For this review, take the finished solid that the model builds, in its own axes (mm). Give positions to 0.01 mm unless a question says otherwise; leave off trailing zeros. Loops run counter-clockwise (first coordinate to the right, second up) from the corner with the lowest first, then second, coordinate; pieces in that order, holes last. Notation, with made-up numbers: (46, 27.5) - (78, 27.5) arc R17 cw to (78, 48.5) - close; hole circle Ø9 at (56, 29). An arc over 180 degrees is marked (long way). Put each result on its own line as item: value.
Autodesk Fusion 360 part; units mm, degrees
sketch "Skizze1" plane through (0, 0, 0) normal (0, 0, 1) x (1, 0, 0)
  line L0 (-2.5, 19.7043) -> (-8.5, 19.7043)
  line L1 (-8.5, 19.7043) -> (-8.5, -52.5)
  line L2 (-8.5, -52.5) -> (-2.5, -52.5)
  line L3 (-2.5, -52.5) -> (-2.5, -35.8)
  line L4 (-2.5, -35.8) -> (0, -38.3)
  line L5 (0, -38.3) -> (0, 38.3)
  line L6 (0, 38.3) -> (-2.5, 35.8)
  line L7 (-2.5, 35.8) -> (-2.5, 19.7043)
  line L8 (-2.5, 35.8) -> (-8.5, 29.8)
  line L9 (-8.5, 29.8) -> (-8.5, 19.7043)
  line L10 (-0.5, 37.8) -> (-0.25, 37.8)
  line L11 (-0.25, 37.8) -> (0, 37.55)
  line L12 (0, 0) -> (7.5514, 0) construction
  line L13 (-0.5, -37.8) -> (-0.25, -37.8)
  line L14 (-0.25, -37.8) -> (0, -37.55)
  dimension "d1" = 45
  dimension "d2" = 2.5
  dimension "d6" = 52.5
  dimension "d31" = 8.5
  dimension "d33" = 16.7
  dimension "d34" = 0.25
  dimension "d36" = 0.25
  dimension "d37" = 82.3
extrude "Extrusion1" add sketch "Skizze1" along normal blind 76 contours L0 L1 L2 L3 L4 L5 L6 L7 L10 L11 L13 L14 | L0 L7 L8 L9
sketch "Skizze2" plane through (0, 0, 0) normal (1, 0, 0) x (0, 1, 0)
  line L0 (-37.55, 0) -> (37.55, 0)
  line L1 (37.55, 76) -> (-37.55, 76)
  line L2 (0, 38) -> (-32.5, 38) construction
  circle A0 centre (-12.5, 38) radius 2
  circle A1 centre (-32.5, 38) radius 2
  circle A2 centre (-22.5, 48) radius 2
  circle A3 centre (-22.5, 28) radius 2
  line L3 (-32.5, 38) -> (-12.5, 38) construction
  line L4 (-22.5, 38) -> (-22.5, 48) construction
  circle A4 centre (-22.5, 38) radius 2
  circle A5 centre (-12.5, 38) radius 3.75
  circle A6 centre (-22.5, 48) radius 3.75
  circle A7 centre (-22.5, 28) radius 3.75
  circle A8 centre (-32.5, 38) radius 3.75
  circle A9 centre (-22.5, 38) radius 3.75
  line L5 (37.55, 0) -> (37.55, 76)
  line L6 (-37.55, 76) -> (-37.55, 0)
  line L7 (0, 76) -> (0, 0) construction
  dimension "d9" = 4
  dimension "d11" = 4
  dimension "d12" = 4
  dimension "d13" = 4
  dimension "d14" = 20
  dimension "d15" = 10
  dimension "d16" = 4
  dimension "d19" = 7.5
  dimension "d20" = 7.5
  dimension "d21" = 7.5
  dimension "d22" = 7.5
  dimension "d23" = 7.5
  dimension "d32" = 12.5
extrude "Extrusion3" cut sketch "Skizze2" against normal blind 4.5 contours A5 | A6 | A7 | A8 | A9
extrude "Extrusion2" cut sketch "Skizze2" against normal up to surface (8.5 mm away) contours A0 | A1 | A2 | A3 | A4
equation "d6 = 12.5 mm + 20 mm + 20 mm"
equation "d11 = d9"
equation "d12 = d9"
equation "d13 = d9"
equation "d16 = d9"
equation "d20 = d19"
equation "d21 = d19"
equation "d22 = d19"
equation "d23 = d19"
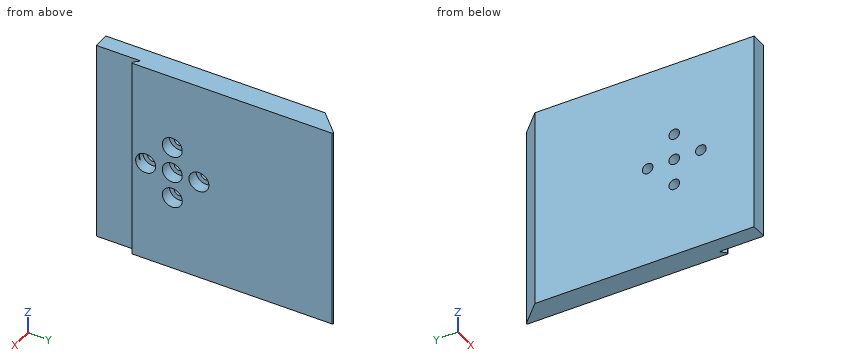
1) Take a section at C-C on y = -12.5. State the section outline as (x, z) points.
Geometry check:
outline: (-8.5, 0) - (0, 0) - (0, 34.25) - (-4.5, 34.25) - (-4.5, 36) - (-8.5, 36) - close; (-8.5, 40) - (-4.5, 40) - (-4.5, 41.75) - (0, 41.75) - (0, 76) - (-8.5, 76) - close
2) Wall thickness on line 1 (Z direction, x = -7, y = -22.5); line 2 (Z direction, x = -2.95, y = -22.5); line 3 (Z direction, x = -6.45, y = -12.5): over which ranges is each line inside the solid? List them lowest first.
Geometry check:
line 1: z = 0 to 26, 30 to 36, 40 to 46, 50 to 76
line 2: z = 0 to 24.25, 31.75 to 34.25, 41.75 to 44.25, 51.75 to 76
line 3: z = 0 to 36, 40 to 76
3) Insertion check: pin 1 Ø5 at (x, z) = (-6.5, 55) entering from +Y; pin 2 Ø2 at (x, z) = (-3.5, 51.5) entering from +Y; pin 3 Ø4.5 at (y, z) = (-12.5, 38) entering from +X. Each pin has a flat end and moves straight along its axis. Give the tip position at first contact, or say it passes through.
Geometry check:
pin 1: stops at y = 34.3
pin 2: stops at y = 35.8
pin 3: stops at x = -4.5
4) Take a section at D-D on z = 38. State how many separate pieces and enclosed holes the cut face has, and give its area (3 significant figures).
Geometry check:
separate pieces: 5
enclosed holes: 0
area: 548 mm²
5) Take a section at A-A on z = 28. State the section outline as (x, y) points, and give its area (3 significant figures).
Geometry check:
outline: (-8.5, -52.5) - (-2.5, -52.5) - (-2.5, -35.8) - (-0.5, -37.8) - (-0.25, -37.8) - (0, -37.55) - (0, -26.25) - (-4.5, -26.25) - (-4.5, -24.5) - (-8.5, -24.5) - close; (-8.5, -20.5) - (-4.5, -20.5) - (-4.5, -18.75) - (0, -18.75) - (0, 37.55) - (-0.25, 37.8) - (-0.5, 37.8) - (-8.5, 29.8) - close
area: 647 mm²
6) Take a section at B-B on y = -22.5. State the section outline as (x, z) points.
Geometry check:
outline: (-8.5, 0) - (0, 0) - (0, 24.25) - (-4.5, 24.25) - (-4.5, 26) - (-8.5, 26) - close; (-8.5, 30) - (-4.5, 30) - (-4.5, 31.75) - (0, 31.75) - (0, 34.25) - (-4.5, 34.25) - (-4.5, 36) - (-8.5, 36) - close; (-8.5, 40) - (-4.5, 40) - (-4.5, 41.75) - (0, 41.75) - (0, 44.25) - (-4.5, 44.25) - (-4.5, 46) - (-8.5, 46) - close; (-8.5, 50) - (-4.5, 50) - (-4.5, 51.75) - (0, 51.75) - (0, 76) - (-8.5, 76) - close
